```python
from build123d import *

# Parameters (mm, degrees)
EXTRUDE_1_DEPTH      = 3
SKETCH_2_W           = 15
SKETCH_2_H           = 3
EXTRUDE_2_DEPTH      = 0.5
FILLET_4_R           = 0.5
SKETCH_6_W           = 118.474287265
SKETCH_6_H           = 3
CUT_EXTRUDE_3_DEPTH  = 10
SKETCH_10_R          = 1.5
CUT_EXTRUDE_7_DEPTH  = 191.555825154
SKETCH_11_R          = 1.5
CUT_EXTRUDE_8_DEPTH  = 191.555825154
SKETCH_15_W          = 15
SKETCH_15_H          = 9
EXTRUDE_4_DEPTH      = 3
FILLET_7_R           = 1
SKETCH_16_R          = 1.5
CUT_EXTRUDE_9_DEPTH  = 194.047828552
EXTRUDE_5_DEPTH      = 3
CUT_EXTRUDE_10_DEPTH = 10
FILLET_8_R           = 2
SKETCH_19_W          = 19.175712735
SKETCH_19_H          = 3
CUT_EXTRUDE_11_DEPTH = 10
FILLET_9_R           = 2
SKETCH_20_W          = 11.767330379
SKETCH_20_H          = 3.399854124
EXTRUDE_6_DEPTH      = 3
SKETCH_21_R          = 1.5
CUT_EXTRUDE_12_DEPTH = 10
SKETCH_23_R          = 1.5
CUT_EXTRUDE_13_DEPTH = 10


with BuildPart() as part:
    # 草图1 → 凸台-拉伸1 (new body)
    with BuildSketch(Plane.XY):
        Polygon((0, 101), (0, 0), (157.65, 0), (157.65, 101), (152.65, 101), (152.65, 107), (137.65, 107), (137.65, 101), (20, 101), (20, 104), (5, 104), (5, 101), align=None)
    extrude(amount=EXTRUDE_1_DEPTH)

    # 草图2 → 凸台-拉伸2 (add)
    with BuildSketch(Plane(origin=(0, 104, 0), x_dir=(1, 0, 0), z_dir=(0, 1, 0))):
        with Locations((12.5, -1.5)):
            Rectangle(SKETCH_2_W, SKETCH_2_H)
    extrude(amount=EXTRUDE_2_DEPTH)

    # 圆角4
    fillet_4_edges = [part.edges().sort_by_distance(p)[0] for p in [
        (0, 0, 1.5),
    ]]
    fillet(fillet_4_edges, radius=FILLET_4_R)

    # 草图6 → 切除-拉伸3 (cut)
    with BuildSketch(Plane.XY.offset(3)):
        with BuildLine():
            Line((5, 3), (0, 3))
            Line((0, 3), (0, 0.5))
            ThreePointArc((0, 0.5), (0.146446609, 0.146446609), (0.5, 0))
            Line((0.5, 0), (5, 0))
            Line((5, 0), (5, 3))
        make_face()
        with Locations((79.237143633, 1.5)):
            Rectangle(SKETCH_6_W, SKETCH_6_H)
    extrude(amount=-CUT_EXTRUDE_3_DEPTH, mode=Mode.SUBTRACT)

    # 草图10 → 切除-拉伸7 (cut, through all)
    with BuildSketch(Plane(origin=(0, 0, 0), x_dir=(-1, 0, 0), z_dir=(0, 0, -1))):
        with Locations((-21.970523915, 6)):
            Circle(SKETCH_10_R)
        with Locations((-11.970523915, 6)):
            Circle(SKETCH_10_R)
    extrude(amount=-CUT_EXTRUDE_7_DEPTH, mode=Mode.SUBTRACT)

    # 草图11 → 切除-拉伸8 (cut, through all)
    with BuildSketch(Plane(origin=(0, 0, 0), x_dir=(-1, 0, 0), z_dir=(0, 0, -1))):
        with Locations((-128.958696033, 6)):
            Circle(SKETCH_11_R)
        with Locations((-118.958696033, 6)):
            Circle(SKETCH_11_R)
    extrude(amount=-CUT_EXTRUDE_8_DEPTH, mode=Mode.SUBTRACT)

    # 草图15 → 凸台-拉伸4 (add)
    with BuildSketch(Plane(origin=(0, 0, 0), x_dir=(-1, 0, 0), z_dir=(0, 0, -1))):
        with Locations((-12.5, 106.877473525)):
            Rectangle(SKETCH_15_W, SKETCH_15_H)
    extrude(amount=-EXTRUDE_4_DEPTH)

    # 圆角7
    fillet_7_edges = [part.edges().sort_by_distance(p)[0] for p in [
        (5, 111.377473525, 1.5),
        (20, 111.377473525, 1.5),
    ]]
    fillet(fillet_7_edges, radius=FILLET_7_R)

    # 草图16 → 切除-拉伸9 (cut, through all)
    with BuildSketch(Plane.XY.offset(3)):
        with Locations((4.752930025, 98)):
            Circle(SKETCH_16_R)
        with Locations((14.752930025, 98)):
            Circle(SKETCH_16_R)
    extrude(amount=-CUT_EXTRUDE_9_DEPTH, mode=Mode.SUBTRACT)

    # 草图17 → 凸台-拉伸5 (add)
    with BuildSketch(Plane.XY.offset(3)):
        with BuildLine():
            Line((19, 130.377473525), (6, 130.377473525))
            ThreePointArc((6, 130.377473525), (5.292893219, 130.084580306), (5, 129.377473525))
            Line((5, 129.377473525), (5, 110.377473525))
            Line((5, 110.377473525), (20, 110.377473525))
            Line((20, 110.377473525), (20, 129.377473525))
            ThreePointArc((20, 129.377473525), (19.707106781, 130.084580306), (19, 130.377473525))
        make_face()
    extrude(amount=-EXTRUDE_5_DEPTH)

    # 草图18 → 切除-拉伸10 (cut)
    with BuildSketch(Plane(origin=(0, 0, 0), x_dir=(-1, 0, 0), z_dir=(0, 0, -1))):
        with BuildLine():
            Line((-133.418834054, 81.437570997), (-133.418834054, 24.201192967))
            ThreePointArc((-133.418834054, 24.201192967), (-138.928819365, 18.691207656), (-144.438804677, 24.201192967))
            Line((-144.438804677, 24.201192967), (-144.438804677, 81.437570997))
            ThreePointArc((-144.438804677, 81.437570997), (-138.928819365, 86.947556308), (-133.418834054, 81.437570997))
        make_face()
        with BuildLine():
            Line((-114.418834054, 81.437570997), (-114.418834054, 24.201192967))
            ThreePointArc((-114.418834054, 24.201192967), (-119.928819365, 18.691207656), (-125.438804677, 24.201192967))
            Line((-125.438804677, 24.201192967), (-125.438804677, 81.437570997))
            ThreePointArc((-125.438804677, 81.437570997), (-119.928819365, 86.947556308), (-114.418834054, 81.437570997))
        make_face()
        with BuildLine():
            Line((-95.418834054, 81.437570997), (-95.418834054, 24.201192967))
            ThreePointArc((-95.418834054, 24.201192967), (-100.928819365, 18.691207656), (-106.438804677, 24.201192967))
            Line((-106.438804677, 24.201192967), (-106.438804677, 81.437570997))
            ThreePointArc((-106.438804677, 81.437570997), (-100.928819365, 86.947556308), (-95.418834054, 81.437570997))
        make_face()
        with BuildLine():
            Line((-76.418834054, 81.437570997), (-76.418834054, 24.201192967))
            ThreePointArc((-76.418834054, 24.201192967), (-81.928819365, 18.691207656), (-87.438804677, 24.201192967))
            Line((-87.438804677, 24.201192967), (-87.438804677, 81.437570997))
            ThreePointArc((-87.438804677, 81.437570997), (-81.928819365, 86.947556308), (-76.418834054, 81.437570997))
        make_face()
        with BuildLine():
            Line((-57.418834054, 81.437570997), (-57.418834054, 24.201192967))
            ThreePointArc((-57.418834054, 24.201192967), (-62.928819365, 18.691207656), (-68.438804677, 24.201192967))
            Line((-68.438804677, 24.201192967), (-68.438804677, 81.437570997))
            ThreePointArc((-68.438804677, 81.437570997), (-62.928819365, 86.947556308), (-57.418834054, 81.437570997))
        make_face()
        with BuildLine():
            Line((-38.418834054, 81.437570997), (-38.418834054, 24.201192967))
            ThreePointArc((-38.418834054, 24.201192967), (-43.928819365, 18.691207656), (-49.438804677, 24.201192967))
            Line((-49.438804677, 24.201192967), (-49.438804677, 81.437570997))
            ThreePointArc((-49.438804677, 81.437570997), (-43.928819365, 86.947556308), (-38.418834054, 81.437570997))
        make_face()
        with BuildLine():
            Line((-19.418834054, 81.437570997), (-19.418834054, 24.201192967))
            ThreePointArc((-19.418834054, 24.201192967), (-24.928819365, 18.691207656), (-30.438804677, 24.201192967))
            Line((-30.438804677, 24.201192967), (-30.438804677, 81.437570997))
            ThreePointArc((-30.438804677, 81.437570997), (-24.928819365, 86.947556308), (-19.418834054, 81.437570997))
        make_face()
    extrude(amount=-CUT_EXTRUDE_10_DEPTH, mode=Mode.SUBTRACT)

    # 圆角8
    fillet_8_edges = [part.edges().sort_by_distance(p)[0] for p in [
        (157.65, 101, 1.5),
        (0, 101, 1.5),
        (137.65, 107, 1.5),
        (152.65, 107, 1.5),
        (0, 3, 1.5),
    ]]
    fillet(fillet_8_edges, radius=FILLET_8_R)

    # 草图19 → 切除-拉伸11 (cut)
    with BuildSketch(Plane.XY.offset(3)):
        with Locations((148.062143633, 1.5)):
            Rectangle(SKETCH_19_W, SKETCH_19_H)
    extrude(amount=-CUT_EXTRUDE_11_DEPTH, mode=Mode.SUBTRACT)

    # 圆角9
    fillet_9_edges = [part.edges().sort_by_distance(p)[0] for p in [
        (157.65, 3, 1.5),
    ]]
    fillet(fillet_9_edges, radius=FILLET_9_R)

    # 草图20 → 凸台-拉伸6 (add)
    with BuildSketch(Plane.XY.offset(3)):
        with Locations((131.393642897, 1.300072938)):
            Rectangle(SKETCH_20_W, SKETCH_20_H)
    extrude(amount=-EXTRUDE_6_DEPTH)

    # 草图21 → 切除-拉伸12 (cut)
    with BuildSketch(Plane(origin=(0, 0, 0), x_dir=(-1, 0, 0), z_dir=(0, 0, -1))):
        with Locations((-12.5, 127.377473525)):
            Circle(SKETCH_21_R)
        with Locations((-12.5, 118.377473525)):
            Circle(SKETCH_21_R)
    extrude(amount=-CUT_EXTRUDE_12_DEPTH, mode=Mode.SUBTRACT)

    # 草图23 → 切除-拉伸13 (cut)
    with BuildSketch(Plane.XY.offset(3)):
        with Locations((148.09274498, 98)):
            Circle(SKETCH_23_R)
        with Locations((138.09274498, 98)):
            Circle(SKETCH_23_R)
    extrude(amount=-CUT_EXTRUDE_13_DEPTH, mode=Mode.SUBTRACT)


solid = part.part
```
Build history of the part. All positions in model axes, mm. A direction names the side the tool comes from. Give positions to 0.01 mm unless a question says otherwise; leave off trailing zeros. One line per question, with ' | ' between items. Start each with the question number.
1) Cut at A-A (y = 41). Count the separate pieces of the cut face and the enclosed holes in it, plus the area to 3 significant figures.
2) 3-axis set-ups, long thin cutter, end or side, ignore diameter. For faces 4 (the flat face through (95, 51, 0)), 5 (the cylindrical face through (120.05, 86.946, 1.479)): which of +Z, -Z, +X, -X, +Y, -Y reach the whole face in a straight line?
3) Two-plate mould, pull along X, no slides. Class faces 1 (the flat face through (95, 51, 3)), 2 (the cylindrical face through (43.808, 18.693, 1.479)), 3 (the cylindrical face through (44.05, 86.946, 1.479)): released by +X, released by -X, zero draft, split by the parting line, or undercut.
4) Pin check, flat tips, straight feed: pin 1 (1.5 mm diameter, centred on y = 118, z = 1.5, fed in from -X); pin 2 (1.5 mm diameter, centred on x = 48.5, y = 57, fed in from -Z); pin 3 (1 mm diameter, centred on x = 45, y = 100.5, fed in from -Z); pin 4 (1.5 mm diameter, centred on x = 148.5, z = 2, fed in from -Y). Stop position of each tip, or through.
5) Probe L1, parallel to Y at x = 22, z = 0.3; L2, parallel to Y at x = 12.5, z = 2.2; L3, parallel to Y at x = 44.5, z = 2.6. List the from-to ranges inside material, lowest first.
Return value:
1) separate pieces: 8 | enclosed holes: 0 | area: 242 mm^2
2) face 4: -Z, +X, -X, +Y, -Y | face 5: +Z, -Z
3) face 1: zero draft | face 2: undercut | face 3: undercut
4) pin 1: x = 5 | pin 2: through | pin 3: z = 0 | pin 4: y = 3
5) L1: 3 to 4.5, 7.5 to 19.53, 86.1 to 101 | L2: 0 to 4.6, 7.4 to 116.88, 119.88 to 125.88, 128.88 to 130.38 | L3: 3 to 18.72, 86.92 to 101
